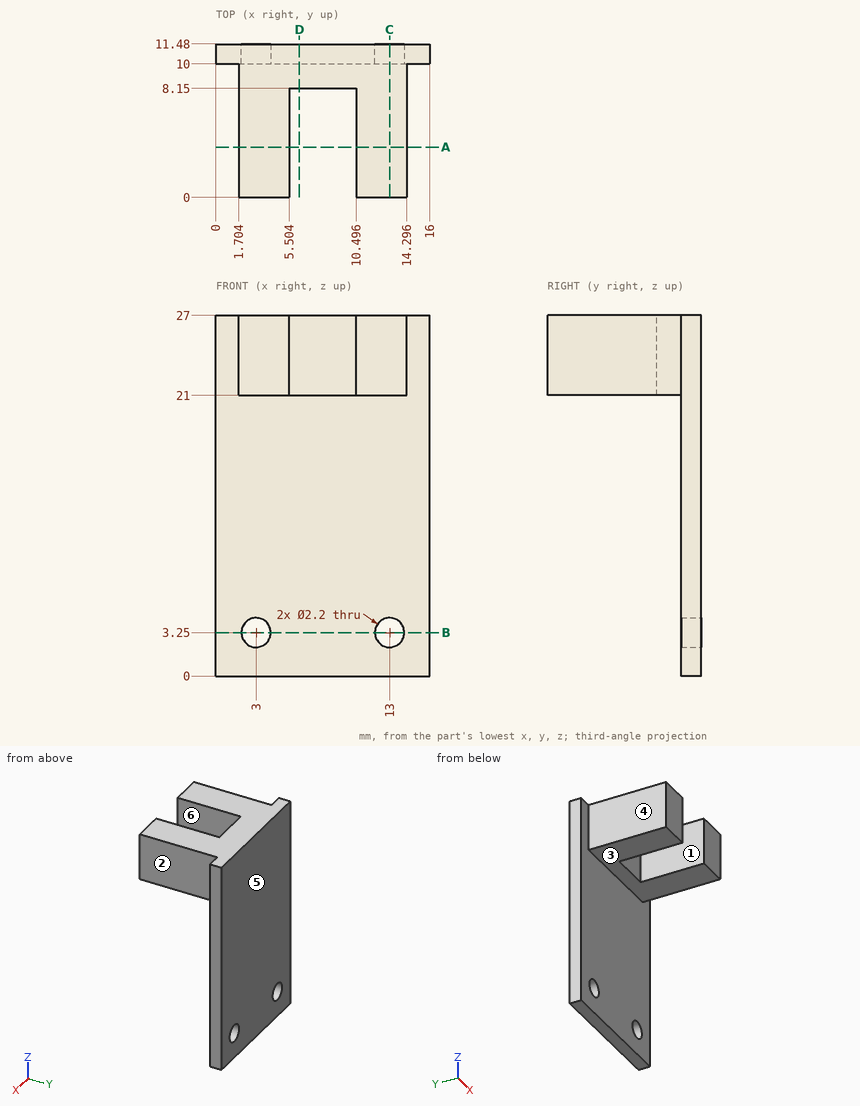
The drawing under review shows one solid part. Ordinate dimensions are in mm from its lowest x, y, z. A direction names the side the tool comes from. Coordinates: 2 decimals unless noted, no trailing zeros. Write each loop counter-clockwise with the first axis right and the second up, starting at its lowest first coordinate (ties: lowest second). Pieces come first, ordered by that corner, then holes. Notation, with made-up numbers: M 8,47.5 L 30,47.5 A5 cw 30,54.5 Z; hole C -16.5,34 d1. An arc over 180 degrees is marked long. Answer as a JSON object with one key per item and string values.
Item 1: Add section A-A, the plane y = 3.75. Give the boundary of the cut face in (x, z), and give its area (3 significant figures).
Outcome:
{"outline": "M 1.7,21 L 5.5,21 L 5.5,27 L 1.7,27 Z; M 10.5,21 L 14.3,21 L 14.3,27 L 10.5,27 Z", "area": "45.6 mm²"}
Item 2: Wall thickness on probe 1 along Z at (x, y) = (13, 11); probe 2 along X at (y, z) = (7.25, 25.75); probe 3 along Z at (x, y) = (3.5, 6.5): over which ranges is each line inside the solid? List them lowest first.
Outcome:
{"probe 1": "0 to 2.15, 4.35 to 27", "probe 2": "1.7 to 5.5, 10.5 to 14.3", "probe 3": "21 to 27"}
Item 3: Add section B-B, the plane z = 3.25. Give the boundary of the cut face in (x, y).
Outcome:
{"outline": "M 0,10 L 1.9,10 L 1.9,11.48 L 0,11.48 Z; M 4.1,10 L 11.9,10 L 11.9,11.48 L 4.1,11.48 Z; M 14.1,10 L 16,10 L 16,11.48 L 14.1,11.48 Z"}
Item 4: Add section D-D, the plane x = 6.25. Give the boundary of the cut face in (y, z).
Outcome:
{"outline": "M 8.15,21 L 10,21 L 10,0 L 11.48,0 L 11.48,27 L 8.15,27 Z"}
Item 5: Draft analysis for pull direction X (two halves, no side actions). For the marked faces 1, 2 and 3, state which applies: pulls with the +X half, pulls with the -X half, needs draft (parallel to the pull), parting line crosses it, or undercut.
Outcome:
{"face 1": "undercut", "face 2": "pulls with the +X half", "face 3": "needs draft"}
Item 6: Insertion check: pin 1 Ø1.8 at (y, z) = (7.5, 23.5) entering from -X; pin 2 Ø3 at (y, z) = (4, 23.5) entering from +X; pin 3 Ø8 at (x, z) = (7.5, 10.5) entering from -Y. Each pin has a flat end and moves straight along its axis. Give the tip position at first contact, or say it passes through.
Outcome:
{"pin 1": "x = 1.7", "pin 2": "x = 14.3", "pin 3": "y = 10"}
Item 7: Machinability: for the marked faces 4, 5 and 6, which of the approach directions +Z, -Z, +X, -X, +Y, -Y give a long, thin tool a straight path to every point of the face, cutting with its end or side? Answer none if there is none.
Outcome:
{"face 4": "+Z, -Z, -X, -Y", "face 5": "+Z, -Z, +X, -X, +Y", "face 6": "+Z, -Z, -Y"}
Item 8: Add section C-C, the plane x = 13. Give the boundary of the cut face in (y, z).
Outcome:
{"outline": "M 0,21 L 10,21 L 10,4.35 L 11.48,4.35 L 11.48,27 L 0,27 Z; M 10,0 L 11.48,0 L 11.48,2.15 L 10,2.15 Z"}
